from build123d import *

# Parameters (mm, degrees)
CUT_EXTRUDE1_DEPTH       = 23.978250743
FILLET1_R                = 1
CIRPATTERN1_COUNT        = 4
FILLET1_OF_CIRPATTERN1_R = 1
SKETCH4_W                = 1
SKETCH4_H                = 0.75
SKETCH9_R                = 1
CUT_EXTRUDE4_DEPTH       = 24.173260612
CIRPATTERN3_COUNT        = 4


with BuildPart() as part:
    # Sketch1 → Revolve1 (revolve)
    with BuildSketch(Plane(origin=(0, 0, 0), x_dir=(1, 0, 0), z_dir=(0, 1, 0)), mode=Mode.PRIVATE) as revolve1_sk:
        Polygon((0, 2.28), (0, 16), (5, 16), (5, 14), (4, 14), (4, 4), (5, 4), (5, 2.28), align=None)
    revolve(revolve1_sk.sketch.rotate(Axis((0, 0, 0), (1, 0, 0)), 180), axis=Axis((0, 0, 0), (1, 0, 0)))

    # Sketch2 → Cut-Revolve1 (revolve, cut)
    with BuildSketch(Plane(origin=(0, 0, 0), x_dir=(1, 0, 0), z_dir=(0, 1, 0))):
        Polygon((2, 0), (2, 16), (2.75, 16), (2.75, 11.5), (2.4, 11.5), (2.4, 0), align=None)
    revolve(axis=Axis((2, 0, 0), (0, 0, -1)), mode=Mode.SUBTRACT)

    # Sketch3 → Cut-Extrude1 (cut, through all)
    with BuildSketch(Plane(origin=(4, 0, 0), x_dir=(0, 0, -1), z_dir=(1, 0, 0))):
        with BuildLine():
            Line((5.196152423, 3), (10.392304845, 6))
            ThreePointArc((10.392304845, 6), (12, 0), (10.392304845, -6))
            Line((10.392304845, -6), (5.196152423, -3))
            ThreePointArc((5.196152423, -3), (6, 0), (5.196152423, 3))
        make_face()
    cut_extrude1 = extrude(amount=-CUT_EXTRUDE1_DEPTH, mode=Mode.SUBTRACT)

    # Fillet1
    fillet1_edges = [part.edges().sort_by_distance(p)[0] for p in [
        (2, -3, -5.196152423),
        (2, 6, -10.392304845),
        (2, -6, -10.392304845),
        (2, 3, -5.196152423),
    ]]
    fillet(fillet1_edges, radius=FILLET1_R)

    # CirPattern1: Cut-Extrude1 ×4 about axis
    cirpattern1_axis = Axis((0, 0, 0), (1, 0, 0))
    for i in range(1, CIRPATTERN1_COUNT):
        add(cut_extrude1.rotate(cirpattern1_axis, i * 360 / CIRPATTERN1_COUNT), mode=Mode.SUBTRACT)

    # Fillet1 of CirPattern1
    fillet1_of_cirpattern1_edges = [part.edges().sort_by_distance(p)[0] for p in [
        (2, 5.196152423, -3),
        (2, 10.392304845, 6),
        (2, 10.392304845, -6),
        (2, 5.196152423, 3),
        (2, 3, 5.196152423),
        (2, -6, 10.392304845),
        (2, 6, 10.392304845),
        (2, -3, 5.196152423),
        (2, -5.196152423, 3),
        (2, -10.392304845, -6),
        (2, -10.392304845, 6),
        (2, -5.196152423, -3),
    ]]
    fillet(fillet1_of_cirpattern1_edges, radius=FILLET1_OF_CIRPATTERN1_R)

    # Sketch4 → Cut-Revolve2 (revolve, cut)
    with BuildSketch(Plane(origin=(0, 0, 0), x_dir=(1, 0, 0), z_dir=(0, 1, 0)), mode=Mode.PRIVATE) as cut_revolve2_sk:
        with Locations((2.5, 15.625)):
            Rectangle(SKETCH4_W, SKETCH4_H)
    revolve(cut_revolve2_sk.sketch.rotate(Axis((0, 0, 0), (1, 0, 0)), 180), axis=Axis((0, 0, 0), (1, 0, 0)), mode=Mode.SUBTRACT)

    # Sketch9 → Cut-Extrude4 (cut, through all)
    with BuildSketch(Plane.ZY):
        with Locations((6.363961031, 6.363961031)):
            Circle(SKETCH9_R)
    cut_extrude4 = extrude(amount=-CUT_EXTRUDE4_DEPTH, mode=Mode.SUBTRACT)

    # CirPattern3: Cut-Extrude4 ×4 about axis
    cirpattern3_axis = Axis((0, 0, 0), (1, 0, 0))
    for i in range(1, CIRPATTERN3_COUNT):
        add(cut_extrude4.rotate(cirpattern3_axis, i * 360 / CIRPATTERN3_COUNT), mode=Mode.SUBTRACT)


solid = part.part
The model under review builds one solid part; all positions refer to its coordinate system, in mm. A direction names the side the tool comes from. Give positions to 0.01 mm unless a question says otherwise; leave off trailing zeros. Loops run counter-clockwise (first coordinate to the right, second up) from the corner with the lowest first, then second, coordinate; pieces in that order, holes last. Notation, with made-up numbers: (56.25, 7) -> (73.25, 7) arc R26 ccw to (73.25, 40) -> close; hole circle Ø9 at (55.25, 2). An arc over 180 degrees is marked (long way). Answer as a JSON object with one key per item and string values. Group by question number.
Q1. Take a section at B-B (y = 8.5). Write out the cut boundary in (x, z), plus the area to 3 significant figures.
Q2. Take a section at A-A (z = 0). State how many separate pieces and enclosed holes the cut face has, plus the area to 3 significant figures.
Q3. Tool access review of faces 1 (the flat face through (4, 3, 3)), 2 (the cylindrical face through (1.25, -0.03, -13.96)), 3 (the cylindrical face through (1.972, -5.552, -2.916)): name each direction out of +Z, -Z, +X, -X, +Y, -Y from which nothing blocks a thin tool from reaching the whole face with its end or side.
Q4. Take a section at C-C (z = 9). Write out the cut boundary in (x, y), plus the area to 3 significant figures.
Q5. Draft analysis for pull direction Z (two halves, no side actions). For faces 4 (the cylindrical face through (1.972, -7.288, 5.981)), 5 (the flat face through (5, 14.15, -0.07)), 6 (the cylindrical face through (2.507, 5.841, 14.087)), 7 (the cylindrical face through (1.97, -5.56, 10.3)), state which applies: pulls with the +Z half, pulls with the -Z half, needs draft (parallel to the pull), parting line crosses it, or undercut.
Q6. Wall thickness on line 1 along X through (y, z) = (13, 9); line 2 along X through (y, z) = (0, -14.3); line 3 along Y through (x, z) = (4.45, 0): over which ranges is each line inside the solid? List them lowest first.
Q7. Insertion check: pin 1 (1.6 mm diameter, centred on y = -6.36, z = -6.36, fed in from +X); pin 2 (1 mm diameter, centred on y = -12.5, z = -1, fed in from +X); pin 3 (1 mm diameter, centred on x = 1.5, z = 4, fed in from -Y). Each pin has a flat end and moves straight along its axis. Give the tip position at first contact, or say it passes through.
Answer below:
{
 "1": {"outline": "(0, -13.56) -> (2, -13.56) -> (2, -12.66) -> (3, -12.66) -> (3, -13.56) -> (5, -13.56) -> (5, -11.12) -> (4, -11.12) -> (4, -4.91) -> (0, -4.91) -> close; (0, 4.91) -> (4, 4.91) -> (4, 11.12) -> (5, 11.12) -> (5, 13.56) -> (3, 13.56) -> (3, 12.66) -> (2, 12.66) -> (2, 13.56) -> (0, 13.56) -> close", "area": "72.3 mm2"},
 "2": {"separate pieces": "4", "enclosed holes": "0", "area": "67.7 mm2"},
 "3": {"face 1": "+X", "face 2": "-Z", "face 3": "+X, -X"},
 "4": {"outline": "(0, -13.23) -> (2, -13.23) -> (2, -12.31) -> (3, -12.31) -> (3, -13.23) -> (5, -13.23) -> (5, -10.72) -> (4, -10.72) -> (4, -5.2) -> (0, -5.2) -> close; (0, 5.2) -> (4, 5.2) -> (4, 10.72) -> (5, 10.72) -> (5, 13.23) -> (3, 13.23) -> (3, 12.31) -> (2, 12.31) -> (2, 13.23) -> (0, 13.23) -> close", "area": "67.4 mm2"},
 "5": {"face 4": "undercut", "face 5": "needs draft", "face 6": "parting line crosses it", "face 7": "undercut"},
 "6": {"line 1": "x = 0 to 2, 3 to 5", "line 2": "x = 0 to 1.25, 2.75 to 5", "line 3": "y = -16 to -14, -4 to -2.28, 2.28 to 4, 14 to 16"},
 "7": {"pin 1": "passes through", "pin 2": "stops at x = 4", "pin 3": "stops at y = -15.61"}
}
